Design review of the part shown in the three views and the two pictorial views. Dimensions are in mm from the part's minimum x, y and z. Coordinates: 2 decimals unless noted, no trailing zeros. Order: outer loops, then holes, each group sorted by start corner. A loop starts at its lowest first (then second) coordinate and runs counter-clockwise, first axis right, second up. Notation, with made-up numbers: M 68.5,49.25 L 117.5,49.25 A16 ccw 117.5,70.25 Z; hole C 67.25,73.25 d9. An arc over 180 degrees is marked long. Use CSV: the item, a comma, the result in double quotes.
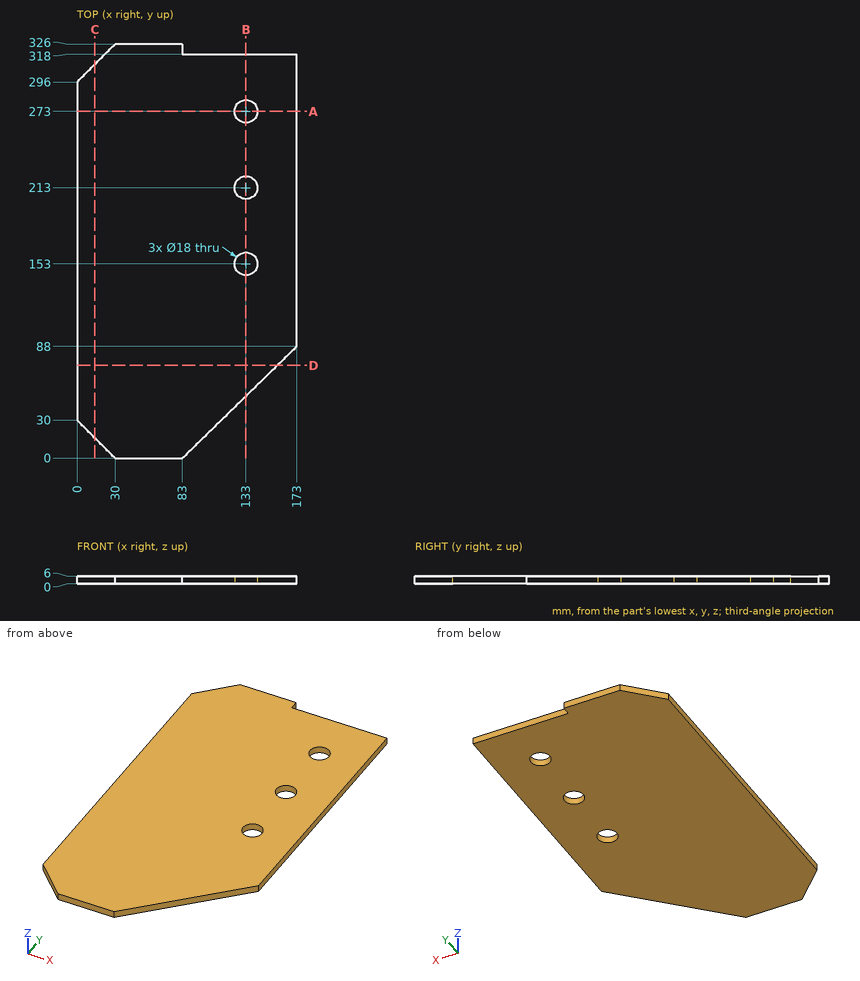
(1) Add section C-C on x = 14. State the section outline as (y, z) points.
The answers:
outline,"M 16,0 L 310,0 L 310,6 L 16,6 Z"
(2) Add section A-A on y = 273. State the section outline as (x, z) points.
The answers:
outline,"M 0,0 L 124,0 L 124,6 L 0,6 Z; M 142,0 L 173,0 L 173,6 L 142,6 Z"
(3) Add section B-B on x = 133. State the section outline as (y, z) points, and give its area (3 significant figures).
The answers:
outline,"M 48.89,0 L 144,0 L 144,6 L 48.89,6 Z; M 162,0 L 204,0 L 204,6 L 162,6 Z; M 222,0 L 264,0 L 264,6 L 222,6 Z; M 282,0 L 318,0 L 318,6 L 282,6 Z"
area,"1,290 mm2"
(4) Add section D-D on y = 73. State the section outline as (x, z) points.
The answers:
outline,"M 0,0 L 157.66,0 L 157.66,6 L 0,6 Z"
(5) Wall thickness on probe 1 along X at (y, z) = (153, 2.2); probe 2 along Y at (x, z) = (133, 4); probe 3 along X at (y, z) = (275, 1.2): over which ranges is each line inside the solid? List them lowest first.
The answers:
probe 1,"x = 0 to 124, 142 to 173"
probe 2,"y = 48.89 to 144, 162 to 204, 222 to 264, 282 to 318"
probe 3,"x = 0 to 124.23, 141.77 to 173"
